from build123d import *

# Parameters (mm, degrees)
SKETCH1_R           = 33
BOSS_EXTRUDE1_DEPTH = 8
SKETCH2_W           = 16
SKETCH2_H           = 10.984378813
BOSS_EXTRUDE2_DEPTH = 8
SKETCH3_R           = 3
SKETCH3_R_2         = 5
CUT_EXTRUDE1_DEPTH  = 9


with BuildPart() as part:
    # Sketch1 → Boss-Extrude1 (new body)
    with BuildSketch(Plane(origin=(0, 0, 0), x_dir=(1, 0, 0), z_dir=(0, 1, 0))):
        Circle(SKETCH1_R)
    extrude(amount=BOSS_EXTRUDE1_DEPTH)

    # Sketch2 → Boss-Extrude2 (add)
    with BuildSketch(Plane(origin=(0, 8, 0), x_dir=(1, 0, 0), z_dir=(0, 1, 0))):
        with Locations((0, 37.507810593)):
            Rectangle(SKETCH2_W, SKETCH2_H)
    extrude(amount=-BOSS_EXTRUDE2_DEPTH)

    # Sketch3 → Cut-Extrude1 (cut, through all)
    with BuildSketch(Plane(origin=(0, 8, 0), x_dir=(1, 0, 0), z_dir=(0, 1, 0))):
        with Locations((0, 18)):
            Circle(SKETCH3_R)
        with Locations((-18, 0)):
            Circle(SKETCH3_R_2)
        with Locations((0, -18)):
            Circle(SKETCH3_R)
        with Locations((18, 0)):
            Circle(SKETCH3_R_2)
    extrude(amount=-CUT_EXTRUDE1_DEPTH, mode=Mode.SUBTRACT)


solid = part.part
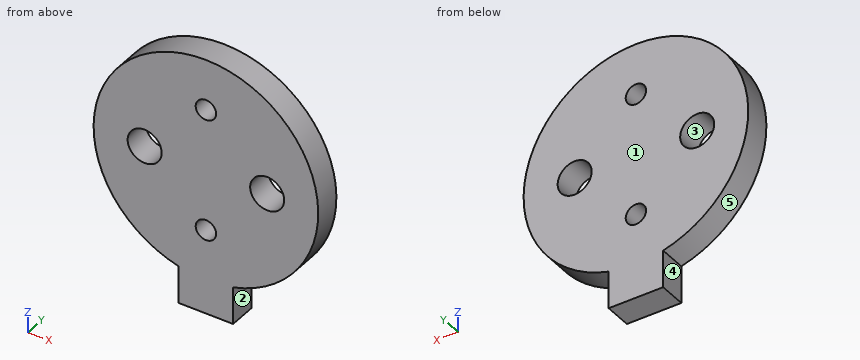
Geometry: final body of the model. Coordinates: model frame, mm. Face numbers are marked on the shaded views. A direction names the side the tool comes from. Give positions to 0.01 mm unless a question says otherwise; leave off trailing zeros. Write each loop counter-clockwise with the first axis right and the second up, starting at its lowest first coordinate (ties: lowest second). Pieces come first, ordered by that corner, then holes.
(1) Ray query, line 1 (Z direction, x = 0, y = 2.5); line 2 (X direction, y = 5.5, z = 0); line 3 (X direction, y = 4, z = 18). Return the intervals inside material, ascending.
(2) First-contact query: P1, Ø3, axis at x = 24.5, y = 7, coming from the +Z side; P2, Ø1.5, axis at x = -15, y = 1.5, coming from the +Z side. Flat tips, straight axial feed; report the tip coordinate or a pass-through.
(3) Cut plane B-B, the plane y = 2.5. Return loops of the section in (x, z).
(4) Cut plane D-D, the plane z = -27. Return loops of the section in (x, y), then the cut area to 3 significant figures.
(5) Mould query, pull axis X, two halves, no side actions, for the marked faces 1, 2 and 3. Classes: released by +X, released by -X, zero draft, split by the parting line, or undercut.
(6) Access query for the marked faces 4 and 5. Directions: +Z, -Z, +X, -X, +Y, -Y. A direction counts if a zero-diameter tool reaches every point of the face in a straight line with its end or side. Return the directions, or none.
(7) Cut plane A-A, the plane x = 18. Return loops of the section in (y, z).
(8) Cut plane C-C, the plane z = -18. Return loops of the section in (x, y).
Values follow:
1. line 1: z = -43 to -21, -15 to 15, 21 to 33
1. line 2: x = -33 to -23, -13 to 13, 23 to 33
1. line 3: x = -27.66 to -3, 3 to 27.66
2. P1: stops at z = 23.66
2. P2: stops at z = 29.76
3. outline: (-8, -43) - (8, -43) - (8, -32.02) arc R33 ccw (long way) to (-8, -32.02) - close; hole circle Ø10 at (-18, 0); hole circle Ø6 at (0, -18); hole circle Ø6 at (0, 18); hole circle Ø10 at (18, 0)
4. outline: (-18.97, 0) - (18.97, 0) - (18.97, 8) - (-18.97, 8) - close
4. area: 304 mm2
5. face 1: zero draft
5. face 2: released by +X
5. face 3: undercut
6. face 4: -Z, -X, +Y, -Y
6. face 5: +Y, -Y
7. outline: (0, -27.66) - (8, -27.66) - (8, -5) - (0, -5) - close; (0, 5) - (8, 5) - (8, 27.66) - (0, 27.66) - close
8. outline: (-27.66, 0) - (-3, 0) - (-3, 8) - (-27.66, 8) - close; (3, 0) - (27.66, 0) - (27.66, 8) - (3, 8) - close
